Can you work these out from the model? Positions are in its coordinate system, mm. Face numbers are marked on the shaded views. Coordinates: 2 decimals unless noted, no trailing zeros. Write each loop counter-clockwise with the first axis right and the second up, starting at its lowest first coordinate (ties: lowest second). Pieces come first, ordered by that corner, then holes. Notation, with made-up numbers: (75, 11) -> (90, 11) arc R9 ccw to (90, 26) -> close; hole circle Ø9 at (-31, -32). An arc over 180 degrees is marked (long way). Answer as CSV lines item,"result". Start each with the question number.
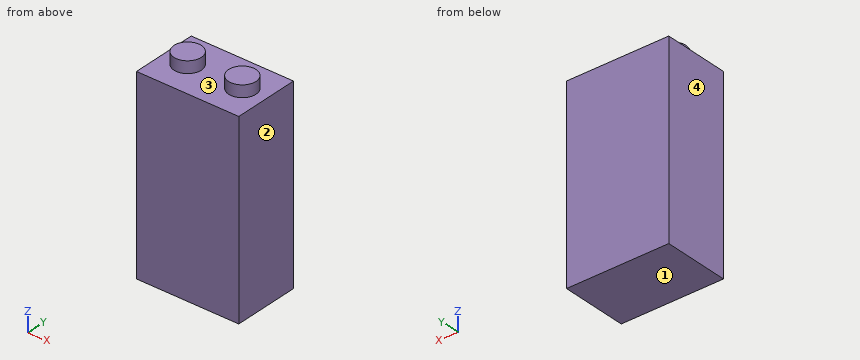
Autodesk Inventor part; units mm, degrees
ref_plane "YZ Plane" through (0, 0, 0) normal (1, 0, 0) x (0, 1, 0)
ref_plane "XZ Plane" through (0, 0, 0) normal (0, 1, 0) x (-1, 0, 0)
ref_plane "XY Plane" through (0, 0, 0) normal (0, 0, 1) x (1, 0, 0)
sketch "Skizze1" plane through (0, 0, 0) normal (0, 1, 0) x (-1, 0, 0)
  line L0 (24.1361, 0) -> (-12.5439, 0)
  line L1 (0, -33.95) -> (0, 33.95)
  line L2 (-7.3039, 24.25) -> (18.8961, 24.25)
  line L3 (18.8961, 24.25) -> (18.8961, -24.25)
  line L4 (18.8961, -24.25) -> (-7.3039, -24.25)
  line L5 (-7.3039, -24.25) -> (-7.3039, 24.25)
  point P0 (0, 0)
  dimension "d0" = 48.5
  dimension "d1" = 26.2
extrude "Extrusion1" add sketch "Skizze1" along normal blind 17
sketch "Skizze3" plane through (-18.8961, 0, 24.25) normal (0, 0, 1) x (1, 0, 0)
  line L0 (26.2, 0) -> (0, 0)
  line L1 (0, 0) -> (0, 17)
  line L2 (0, 17) -> (26.2, 17)
  line L3 (13.1, 17) -> (13.1, 0)
  circle A0 centre (6.1, 8.5) radius 3.5
  circle A1 centre (20.1, 8.5) radius 3.5
  point P0 (18.8961, 0)
  dimension "d7" = 13.1
  dimension "d8" = 7
  dimension "d9" = 8.5
  dimension "d10" = 7
extrude "Extrusion2" add sketch "Skizze3" along normal blind 3 contours A0 | A1
equation "\"d10\" = usedParameter"
equation "\"usedParameter\" = 7"
equation "\"unusedParameter\" = 42"
properties part number "9VBatterie_2017only" material "Edelstahl"
Q1. Imagine slicing it at B-B (x = -15.25). Write out the boundary of the cut face in (y, z).
Q2. Imagine slicing it at A-A (y = 8.5). Write out the boundary of the cut face in (x, z), then the cut area to 3 significant figures.
Q3. Imagine slicing it at C-C (y = 14.5). Write out the boundary of the cut face in (x, z).
Q4. For pin 1 (4 mm diameter, centred on x = -4, y = 11, fed in from +Z), with a flat end and sliding along its axis, tell me the tip position at first contact or that it passes through.
Q5. If we mould it in two halves opening along X, with no side actions, what happens to the marked faces 1, 2, 3 and 4? For each: released by +X, released by -X, zero draft, split by the parting line, or undercut.
Q6. Imagine slicing it at D-D (x = 5.75). Write out the boundary of the cut face in (y, z).
Q7. I need wall thicknesses on L1, parallel to Z at x = 5.5, y = 15.5. Which ranges of the line are inside material? Lowest first, please.
Entries:
1,outline,"(0, -24.25) -> (17, -24.25) -> (17, 24.25) -> (11, 24.25) -> (11, 27.25) -> (6, 27.25) -> (6, 24.25) -> (0, 24.25) -> close"
2,outline,"(-18.9, -24.25) -> (7.3, -24.25) -> (7.3, 24.25) -> (4.7, 24.25) -> (4.7, 27.25) -> (-2.3, 27.25) -> (-2.3, 24.25) -> (-9.3, 24.25) -> (-9.3, 27.25) -> (-16.3, 27.25) -> (-16.3, 24.25) -> (-18.9, 24.25) -> close"
2,area,"1,310 mm2"
3,outline,"(-18.9, -24.25) -> (7.3, -24.25) -> (7.3, 24.25) -> (-18.9, 24.25) -> close"
4,pin 1,"z = 24.25"
5,face 1,"zero draft"
5,face 2,"released by +X"
5,face 3,"undercut"
5,face 4,"released by -X"
6,outline,"(0, -24.25) -> (17, -24.25) -> (17, 24.25) -> (0, 24.25) -> close"
7,L1,"-24.25 to 24.25"
